Can you work these out from the model? Positions are in its coordinate system, mm. A direction names the side the tool comes from. Give positions to 0.01 mm unless a question says otherwise; leave off trailing zeros. Write each loop counter-clockwise with the first axis right and the second up, starting at its lowest first coordinate (ties: lowest second). Pieces come first, ordered by that corner, then holes. Notation, with made-up numbers: (18.25, 60) -> (33.25, 60) arc R37 cw to (33.25, 99) -> close; hole circle Ø10 at (58.25, -8). An arc over 180 degrees is marked (long way). Answer as CSV lines item,"result". Start each with the question number.
1. If we mould it in two halves opening along Z, with no side actions, what happens to faces 1 (the face through (0, 0, 0)), 2 (the face through (3, -2, -2.8)), 3 (the face through (3.9, 1, 0))? For each: pulls with the +Z half, pulls with the -Z half, needs draft (parallel to the pull), parting line crosses it, or undercut.
2. If we section it at B-B on z = -3: Write out the boundary of the cut face in (x, y).
3. If we section it at A-A on y = -0.75: Write out the boundary of the cut face in (x, z), plus the area to 3 significant figures.
4. I'm going to push flat-ended pins straight in: P1, Ø1, axis at x = -1.5, y = -2, coming from the -Z side; P2, Ø0.8, axis at x = 3, y = -2.5, coming from the +Z side; P3, Ø0.8, axis at x = 2.5, y = -1.5, coming from the -Z side; P4, Ø1, axis at x = 0.5, z = 0.5, coming from the -Y side. Where does each tip first touch, or does it pass through?
5. I need wall thicknesses on line 1 (Z direction, x = -2.75, y = -1.75); line 2 (Y direction, x = 3, z = -2.5); line 3 (Y direction, x = 3.5, z = 3.75). Which ranges of each line are inside material? Lowest first, please. Write a range as [from, to].
6. On a 3-axis mill with a long thin cutter (end or side, diameter ignored), from which of +Z, -Z, +X, -X, +Y, -Y can I reach the whole of each face in a straight line? I mean faces 4 (the face through (3, -2, 2.36)), 5 (the face through (1, 2.4, -3)), 6 (the face through (-3, -2, 2.8)), 7 (the face through (-3.4, 1.1, 3.4)), 8 (the face through (-3, -2, -2.8)). Say none if no direction works.
```python
from build123d import *
from build123d.topology import SkipClean

# Parameters (mm, degrees)
EXTRUDE1_DEPTH = 2.4
FILLET1_R      = 0.15
SKETCH3_W      = 1.5
SKETCH3_H      = 0.44
EXTRUDE2_DEPTH = 4.85


with BuildPart() as part:
    # Sketch1 → Extrude1 (new body)
    with BuildSketch(Plane(origin=(0, 0, 0), x_dir=(1, 0, 0), z_dir=(0, 1, 0))):
        Polygon((-2.9, -3.9), (3.9, -3.9), (3.9, 3.9), (-3.9, 3.9), (-3.9, -2.9), align=None)
    extrude(amount=EXTRUDE1_DEPTH)

    # Sketch2 → Revolve1 (revolve)
    with SkipClean():  # the faces are left unmerged after this step: merging them gives an invalid solid
        with BuildSketch(Plane.XY):
            with BuildLine():
                ThreePointArc((0, 4.9), (-1.767766953, 4.167766953), (-2.5, 2.4))
                Line((-2.5, 2.4), (0, 2.4))
                Line((0, 2.4), (0, 4.9))
            make_face()
            with BuildLine():
                Line((0, 4.9), (0, 2.4))
                Line((0, 2.4), (2.5, 2.4))
                ThreePointArc((2.5, 2.4), (1.767766953, 4.167766953), (0, 4.9))
            make_face()
        revolve(axis=Axis((0, 2.4, 0), (0, 1, 0)))
    add(part.part.scale(1), mode=Mode.REPLACE)  # the faces are merged on a copy

    # Fillet1
    fillet1_edges = [part.edges().sort_by_distance(p)[0] for p in [
        (-3.9, 2.4, -0.5),
        (-3.4, 2.4, 3.4),
        (2.5, 2.4, 0),
        (0.5, 2.4, 3.9),
        (3.9, 2.4, 0),
        (0, 2.4, -3.9),
        (3.9, 1.2, 3.9),
        (-2.9, 1.2, 3.9),
        (-3.9, 1.2, 2.9),
        (-3.9, 1.2, -3.9),
        (3.9, 1.2, -3.9),
    ]]
    fillet(fillet1_edges, radius=FILLET1_R)

    # Sketch3 → Extrude2 (add)
    with BuildSketch(Plane.XZ):
        with Locations((-2.85, 2.58)):
            Rectangle(SKETCH3_W, SKETCH3_H)
        with Locations((2.85, 2.58)):
            Rectangle(SKETCH3_W, SKETCH3_H)
        with Locations((2.85, -2.58)):
            Rectangle(SKETCH3_W, SKETCH3_H)
        with Locations((-2.85, -2.58)):
            Rectangle(SKETCH3_W, SKETCH3_H)
    extrude(amount=EXTRUDE2_DEPTH)


solid = part.part
```
Computed values:
1,face 1,"undercut"
1,face 2,"pulls with the -Z half"
1,face 3,"needs draft"
2,outline,"(-3.9, 0) -> (3.9, 0) -> (3.9, 2.25) arc R0.15 ccw to (3.75, 2.4) -> (-3.75, 2.4) arc R0.15 ccw to (-3.9, 2.25) -> close"
3,outline,"(-3.6, -2.8) -> (-2.1, -2.8) -> (-2.1, -2.36) -> (-3.6, -2.36) -> close; (-3.6, 2.36) -> (-2.1, 2.36) -> (-2.1, 2.8) -> (-3.6, 2.8) -> close; (2.1, -2.8) -> (3.6, -2.8) -> (3.6, -2.36) -> (2.1, -2.36) -> close; (2.1, 2.36) -> (3.6, 2.36) -> (3.6, 2.8) -> (2.1, 2.8) -> close"
3,area,"2.64 mm2"
4,P1,"passes through"
4,P2,"stops at z = 2.8"
4,P3,"stops at z = -2.8"
4,P4,"stops at y = 0"
5,line 1,"z = [-2.8, -2.36], [2.36, 2.8]"
5,line 2,"y = [-4.85, 2.4]"
5,line 3,"y = [0, 2.4]"
6,face 4,"+X, -X, -Y"
6,face 5,"+Y"
6,face 6,"+Z, +X, -X, -Y"
6,face 7,"+Z, -X, +Y, -Y"
6,face 8,"-Z, +X, -X, -Y"
